Geometry: final body of the model. Coordinates: model frame, mm. Face numbers are marked on the shaded views. A direction names the side the tool comes from. Round coordinates to 2 decimals unless told otherwise and drop trailing zeros. Loops run counter-clockwise (first coordinate to the right, second up) from the corner with the lowest first, then second, coordinate; pieces in that order, holes last. Notation, with made-up numbers: M 43.5,53.5 L 74.5,53.5 A21 cw 74.5,83.5 Z; hole C -1.75,16.25 d1. An arc over 180 degrees is marked long. Return JSON: item names as keys, results as strings.
from build123d import *
from build123d import SkipClean  # not in build123d's __all__

# Parameters (mm, degrees)
F1_DEPTH = 38.1
F0_R     = 9.525
F2_DEPTH = 19.05
F0_R_2   = 12.7
F3_DEPTH = 19.05
F4_DEPTH = 50.8


with BuildPart() as f1:
    # F0 (on Top) → F1 (new body)
    with BuildSketch(Plane.XY):
        with BuildLine():
            ThreePointArc((6.35, 24.5934442484), (17.9605122421, 17.9605122421), (24.5934442484, 6.35))
            Line((24.5934442484, 6.35), (34.3428758988, 6.35))
            ThreePointArc((34.3428758988, 6.35), (24.6957043329, 24.6957043329), (6.35, 34.3428758988))
            Line((6.35, 34.3428758988), (6.35, 24.5934442484))
        make_face()
        with BuildLine():
            ThreePointArc((-6.35, 24.5934442484), (0, 25.4), (6.35, 24.5934442484))
            Line((6.35, 24.5934442484), (6.35, 34.3428758988))
            ThreePointArc((6.35, 34.3428758988), (0, 34.925), (-6.35, 34.3428758988))
            Line((-6.35, 34.3428758988), (-6.35, 24.5934442484))
        make_face()
        with BuildLine():
            ThreePointArc((-24.5934442484, 6.35), (-17.9605122421, 17.9605122421), (-6.35, 24.5934442484))
            Line((-6.35, 24.5934442484), (-6.35, 34.3428758988))
            ThreePointArc((-6.35, 34.3428758988), (-24.6957043329, 24.6957043329), (-34.3428758988, 6.35))
            Line((-34.3428758988, 6.35), (-24.5934442484, 6.35))
        make_face()
        with BuildLine():
            ThreePointArc((-24.5934442484, -6.35), (-25.4, 0), (-24.5934442484, 6.35))
            Line((-24.5934442484, 6.35), (-34.3428758988, 6.35))
            ThreePointArc((-34.3428758988, 6.35), (-34.925, 0), (-34.3428758988, -6.35))
            Line((-34.3428758988, -6.35), (-24.5934442484, -6.35))
        make_face()
        with BuildLine():
            Line((-6.35, -34.3428758988), (-6.35, -24.5934442484))
            ThreePointArc((-6.35, -24.5934442484), (-17.9605122421, -17.9605122421), (-24.5934442484, -6.35))
            Line((-24.5934442484, -6.35), (-34.3428758988, -6.35))
            ThreePointArc((-34.3428758988, -6.35), (-24.6957043329, -24.6957043329), (-6.35, -34.3428758988))
        make_face()
        with BuildLine():
            Line((6.35, -34.3428758988), (6.35, -24.5934442484))
            ThreePointArc((6.35, -24.5934442484), (0, -25.4), (-6.35, -24.5934442484))
            Line((-6.35, -24.5934442484), (-6.35, -34.3428758988))
            ThreePointArc((-6.35, -34.3428758988), (0, -34.925), (6.35, -34.3428758988))
        make_face()
        with BuildLine():
            Line((34.3428758988, -6.35), (24.5934442484, -6.35))
            ThreePointArc((24.5934442484, -6.35), (17.9605122421, -17.9605122421), (6.35, -24.5934442484))
            Line((6.35, -24.5934442484), (6.35, -34.3428758988))
            ThreePointArc((6.35, -34.3428758988), (24.6957043329, -24.6957043329), (34.3428758988, -6.35))
        make_face()
        with BuildLine():
            ThreePointArc((24.5934442484, 6.35), (25.1975542852, 3.2005090291), (25.4, 0))
            ThreePointArc((25.4, 0), (25.1975542852, -3.2005090291), (24.5934442484, -6.35))
            Line((24.5934442484, -6.35), (34.3428758988, -6.35))
            ThreePointArc((34.3428758988, -6.35), (34.7791644937, -3.1883133656), (34.925, 0))
            ThreePointArc((34.925, 0), (34.7791644937, 3.1883133656), (34.3428758988, 6.35))
            Line((34.3428758988, 6.35), (24.5934442484, 6.35))
        make_face()
    extrude(amount=F1_DEPTH)

    # F0 (on Top) → F2 (join)
    with BuildSketch(Plane.XY):
        with BuildLine():
            Line((-60.3174545175, -16.5021301071), (-21.0389726486, -39.1556398223))
            ThreePointArc((-21.0389726486, -39.1556398223), (0, -44.7878622326), (21.0389726486, -39.1556398223))
            Line((21.0389726486, -39.1556398223), (60.3174545175, -16.5021301071))
            ThreePointArc((60.3174545175, -16.5021301071), (69.8600459872, -0.008704331), (60.3325297632, 16.4934343301))
            Line((60.3325297632, 16.4934343301), (21.0389726486, 39.1556398223))
            ThreePointArc((21.0389726486, 39.1556398223), (0, 44.787862505), (-21.0389726486, 39.1556398223))
            Line((-21.0389726486, 39.1556398223), (-60.332536636, 16.4934343301))
            ThreePointArc((-60.332536636, 16.4934343301), (-69.8600525487, -0.0087063185), (-60.3174545175, -16.5021301071))
        make_face()
        with BuildLine():
            ThreePointArc((6.35, 34.3428758988), (24.6957043329, 24.6957043329), (34.3428758988, 6.35))
            ThreePointArc((34.3428758988, 6.35), (34.7791644937, 3.1883133656), (34.925, 0))
            ThreePointArc((34.925, 0), (34.7791644937, -3.1883133656), (34.3428758988, -6.35))
            ThreePointArc((34.3428758988, -6.35), (24.6957043329, -24.6957043329), (6.35, -34.3428758988))
            ThreePointArc((6.35, -34.3428758988), (0, -34.925), (-6.35, -34.3428758988))
            ThreePointArc((-6.35, -34.3428758988), (-24.6957043329, -24.6957043329), (-34.3428758988, -6.35))
            ThreePointArc((-34.3428758988, -6.35), (-34.925, 0), (-34.3428758988, 6.35))
            ThreePointArc((-34.3428758988, 6.35), (-24.6957043329, 24.6957043329), (-6.35, 34.3428758988))
            ThreePointArc((-6.35, 34.3428758988), (0, 34.925), (6.35, 34.3428758988))
        make_face(mode=Mode.SUBTRACT)
        with Locations((-50.7999965718, 5.9441e-06)):
            Circle(F0_R, mode=Mode.SUBTRACT)
        with Locations((50.7999931345, 3.9617e-06)):
            Circle(F0_R, mode=Mode.SUBTRACT)
    extrude(amount=F2_DEPTH)

    # F0 (on Top) → F3 (join)
    with BuildSketch(Plane.XY):
        with BuildLine():
            ThreePointArc((24.5934442484, -6.35), (25.1975542852, -3.2005090291), (25.4, 0))
            ThreePointArc((25.4, 0), (25.1975542852, 3.2005090291), (24.5934442484, 6.35))
            ThreePointArc((24.5934442484, 6.35), (17.9605122421, 17.9605122421), (6.35, 24.5934442484))
            ThreePointArc((6.35, 24.5934442484), (0, 25.4), (-6.35, 24.5934442484))
            ThreePointArc((-6.35, 24.5934442484), (-17.9605122421, 17.9605122421), (-24.5934442484, 6.35))
            ThreePointArc((-24.5934442484, 6.35), (-25.4, 0), (-24.5934442484, -6.35))
            ThreePointArc((-24.5934442484, -6.35), (-17.9605122421, -17.9605122421), (-6.35, -24.5934442484))
            ThreePointArc((-6.35, -24.5934442484), (0, -25.4), (6.35, -24.5934442484))
            ThreePointArc((6.35, -24.5934442484), (17.9605122421, -17.9605122421), (24.5934442484, -6.35))
        make_face()
        Circle(F0_R_2, mode=Mode.SUBTRACT)
    extrude(amount=F3_DEPTH)

    # F0 (on Top) → F4 (join)
    with BuildSketch(Plane.XY):
        with BuildLine():
            ThreePointArc((-24.5934442484, 6.35), (-17.9605122421, 17.9605122421), (-6.35, 24.5934442484))
            Line((-6.35, 24.5934442484), (-6.35, 34.3428758988))
            ThreePointArc((-6.35, 34.3428758988), (-24.6957043329, 24.6957043329), (-34.3428758988, 6.35))
            Line((-34.3428758988, 6.35), (-24.5934442484, 6.35))
        make_face()
        with BuildLine():
            ThreePointArc((6.35, 24.5934442484), (17.9605122421, 17.9605122421), (24.5934442484, 6.35))
            Line((24.5934442484, 6.35), (34.3428758988, 6.35))
            ThreePointArc((34.3428758988, 6.35), (24.6957043329, 24.6957043329), (6.35, 34.3428758988))
            Line((6.35, 34.3428758988), (6.35, 24.5934442484))
        make_face()
        with BuildLine():
            Line((34.3428758988, -6.35), (24.5934442484, -6.35))
            ThreePointArc((24.5934442484, -6.35), (17.9605122421, -17.9605122421), (6.35, -24.5934442484))
            Line((6.35, -24.5934442484), (6.35, -34.3428758988))
            ThreePointArc((6.35, -34.3428758988), (24.6957043329, -24.6957043329), (34.3428758988, -6.35))
        make_face()
        with BuildLine():
            Line((-6.35, -34.3428758988), (-6.35, -24.5934442484))
            ThreePointArc((-6.35, -24.5934442484), (-17.9605122421, -17.9605122421), (-24.5934442484, -6.35))
            Line((-24.5934442484, -6.35), (-34.3428758988, -6.35))
            ThreePointArc((-34.3428758988, -6.35), (-24.6957043329, -24.6957043329), (-6.35, -34.3428758988))
        make_face()
    with SkipClean():  # cleaning this boolean's faces spoils the solid; the shape is the same uncleaned
        extrude(amount=F4_DEPTH)


solid = f1.part
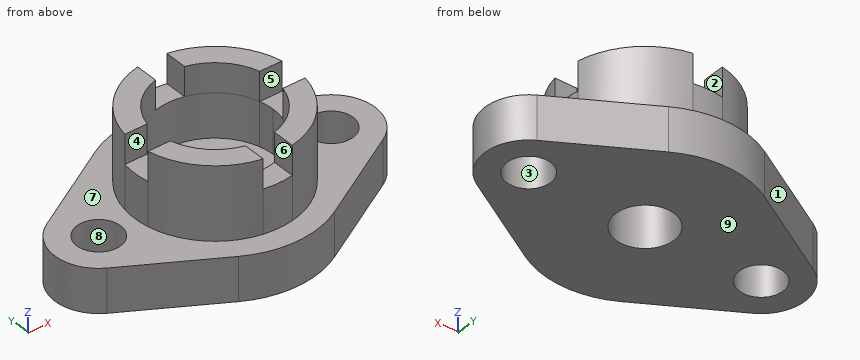
Q1. Pull-direction query (Y, two-part tool) for the marked faces 1, 2, 3 and 4; classes: pulls with the +Y half, pulls with the -Y half, needs draft (parallel to the pull), parting line crosses it, or undercut.
Determined:
{"face 1": "pulls with the +Y half", "face 2": "needs draft", "face 3": "undercut", "face 4": "undercut"}
Q2. Section query B-B (x = 0). Output: boundary loops of the cut face in (y, z) (3 decimals), plus the area to 3 significant figures.
Determined:
{"outline": "M -44.788,0 L -12.7,0 L -12.7,19.05 L -25.4,19.05 L -25.4,38.1 L -34.925,38.1 L -34.925,19.05 L -44.788,19.05 Z; M 12.7,0 L 44.788,0 L 44.788,19.05 L 34.925,19.05 L 34.925,38.1 L 25.4,38.1 L 25.4,19.05 L 12.7,19.05 Z", "area": "1,590 mm^2"}
Q3. Pin query (flat end, axial travel): pin 1 (15 mm diameter, centred on x = 0, y = 0, fed in from +Z); pin 2 (10.5 mm diameter, centred on y = 29, z = 47, fed in from +X); pin 3 (8.5 mm diameter, centred on x = 1.5, y = -30.5, fed in from +Z); pin 4 (3 mm diameter, centred on y = -27, z = 47, fed in from -X). Return the tip coordinate at first contact, or that it passes through.
Determined:
{"pin 1": "passes through", "pin 2": "stops at x = 25.61", "pin 3": "stops at z = 38.1", "pin 4": "stops at x = -23.86"}
Q4. Reachability of the marked faces 5, 6, 7, 8 and 9 from +Z, -Z, +X, -X, +Y, -Y: full face, straight path, thin tool, end or side. Return the list, or none.
Determined:
{"face 5": "+Z, +X, -X", "face 6": "+Z, +Y, -Y", "face 7": "+Z", "face 8": "+Z, -Z", "face 9": "-Z, +X, -X, +Y, -Y"}
Q5. Section query C-C (y = 18). Output: boundary loops of the cut face in (x, z), plus the area to 3 significant figures.
Determined:
{"outline": "M -57.72,0 L 57.72,0 L 57.72,19.05 L 29.93,19.05 L 29.93,50.8 L 17.92,50.8 L 17.92,19.05 L -17.92,19.05 L -17.92,50.8 L -29.93,50.8 L -29.93,19.05 L -57.72,19.05 Z", "area": "2,960 mm^2"}
Q6. Section query A-A (z = 12.5). Output: boundary loops of the cut face in (x, y) (3 decimals), plus the area to 3 significant figures.
Determined:
{"outline": "M -60.333,16.493 A19.04 ccw -60.317,-16.502 L -21.039,-39.156 A42.111 ccw 21.039,-39.156 L 60.317,-16.502 A19.04 ccw 60.333,16.493 L 21.039,39.156 A42.111 ccw -21.039,39.156 Z; hole C -50.8,0 d19.05; hole C 0,0 d25.4; hole C 50.8,0 d19.05", "area": "7,360 mm^2"}
Q7. Section query D-D (x = -30). Output: boundary loops of the cut face in (y, z), plus the area to 3 significant figures.
Determined:
{"outline": "M -33.99,0 L 33.99,0 L 33.99,19.05 L 17.88,19.05 L 17.88,50.8 L 6.35,50.8 L 6.35,38.1 L -6.35,38.1 L -6.35,50.8 L -17.88,50.8 L -17.88,19.05 L -33.99,19.05 Z", "area": "2,270 mm^2"}
Q8. Material intervals for L1, parallel to X at y = -2, z = 4.5; L2, parallel to X at y = -19, z = 19.5; L3, parallel to X at y = -7.5, z = 25, sorted ascending.
Determined:
{"L1": "x = -69.75 to -60.11, -41.49 to -12.54, 12.54 to 41.49, 60.11 to 69.75", "L2": "x = -29.3 to -16.86, 16.86 to 29.3", "L3": "x = -34.11 to -24.27, 24.27 to 34.11"}
